```python
from build123d import *

# Parameters (mm, degrees)
SKETCH1_W           = 42.3
SKETCH1_H           = 42.3
BOSS_EXTRUDE1_DEPTH = 3
SKETCH2_R           = 1.5
CUT_EXTRUDE1_DEPTH  = 4
SKETCH5_W           = 3
SKETCH5_H           = 42.3
BOSS_EXTRUDE2_DEPTH = 40
CUT_EXTRUDE2_DEPTH  = 40
SKETCH7_R           = 1.5
CUT_EXTRUDE3_DEPTH  = 4


with BuildPart() as part:
    # Sketch1 → Boss-Extrude1 (new body)
    with BuildSketch(Plane(origin=(0, 0, 0), x_dir=(1, 0, 0), z_dir=(0, 1, 0))):
        with Locations((21.15, 21.15)):
            Rectangle(SKETCH1_W, SKETCH1_H)
    extrude(amount=BOSS_EXTRUDE1_DEPTH)

    # Sketch2 → Cut-Extrude1 (cut, through all)
    with BuildSketch(Plane(origin=(0, 3, 0), x_dir=(1, 0, 0), z_dir=(0, 1, 0))):
        with Locations((5.65, 5.65)):
            Circle(SKETCH2_R)
        with Locations((36.65, 5.65)):
            Circle(SKETCH2_R)
        with Locations((36.65, 36.65)):
            Circle(SKETCH2_R)
        with Locations((5.65, 36.65)):
            Circle(SKETCH2_R)
    extrude(amount=-CUT_EXTRUDE1_DEPTH, mode=Mode.SUBTRACT)

    # Sketch5 → Boss-Extrude2 (add)
    with BuildSketch(Plane(origin=(0, 3, 0), x_dir=(1, 0, 0), z_dir=(0, 1, 0))):
        with Locations((40.8, 21.15)):
            Rectangle(SKETCH5_W, SKETCH5_H)
    extrude(amount=BOSS_EXTRUDE2_DEPTH)

    # Sketch6 → Cut-Extrude2 (cut)
    with BuildSketch(Plane.ZY.offset(-39.3)):
        Polygon((-42.3, 43), (-22.3, 43), (-42.3, 23), align=None)
    extrude(amount=-CUT_EXTRUDE2_DEPTH, mode=Mode.SUBTRACT)

    # Sketch7 → Cut-Extrude3 (cut, through all)
    with BuildSketch(Plane.ZY.offset(-39.3)):
        with Locations((-10, 33)):
            Circle(SKETCH7_R)
        with Locations((-10, 13)):
            Circle(SKETCH7_R)
    extrude(amount=-CUT_EXTRUDE3_DEPTH, mode=Mode.SUBTRACT)


solid = part.part
```
Can you work these out from the model? Positions are in its coordinate system, mm. A direction names the side the tool comes from. Coordinates: 2 decimals unless noted, no trailing zeros. Order: outer loops, then holes, each group sorted by start corner. A loop starts at its lowest first (then second) coordinate and runs counter-clockwise, first axis right, second up. Notation, with made-up numbers: (13.5, -10.5) - (49.5, -10.5) arc R17 cw to (49.5, 16.5) - close; hole circle Ø8 at (84, 7). An arc over 180 degrees is marked (long way). Answer in a Markdown table with one row per item.
1. Suppose I cut it at C-C (y = 13). Please give me the cut outline in (x, z).
Reply:
| item | result |
|---|---|
| outline | (39.3, -42.3) - (42.3, -42.3) - (42.3, -11.5) - (39.3, -11.5) - close; (39.3, -8.5) - (42.3, -8.5) - (42.3, 0) - (39.3, 0) - close |
2. If we mould it in two halves opening along X, with no side actions, what happens to faces 3 (the flat face through (30, 2, 0)), 4 (the cylindrical face through (38.08, 1.52, -6.1)), 5 (the flat face through (0, 1, -21))? For each: pulls with the +X half, pulls with the -X half, needs draft (parallel to the pull), parting line crosses it, or undercut.
Reply:
| item | result |
|---|---|
| face 3 | needs draft |
| face 4 | undercut |
| face 5 | pulls with the -X half |
3. If I drill on line 1 along Y through (x, z) = (40.4, -10); line 2 along Z through (x, y) = (36.65, 2.25); line 3 along X through (y, z) = (2.3, -5.65), over which ranges is the centre line in solid material (lowest first)?
Reply:
| item | result |
|---|---|
| line 1 | y = 0 to 11.5, 14.5 to 31.5, 34.5 to 43 |
| line 2 | z = -42.3 to -38.15, -35.15 to -7.15, -4.15 to 0 |
| line 3 | x = 0 to 4.15, 7.15 to 35.15, 38.15 to 42.3 |
4. For pin 1 (5 mm diameter, centred on y = 33, z = -10, fed in from +X); pin 2 (4 mm diameter, centred on x = 36.65, z = -36.65, fed in from +Y); pin 3 (10 mm diameter, centred on y = 29.5, z = -15.5, fed in from -X), each with a flat end and sliding along its axis, tell me the tip position at first contact or that it passes through.
Reply:
| item | result |
|---|---|
| pin 1 | stops at x = 42.3 |
| pin 2 | stops at y = 3 |
| pin 3 | stops at x = 39.3 |
5. Suppose I cut it at B-B (x = 36.65). Please give me the cut outline in (y, z).
Reply:
| item | result |
|---|---|
| outline | (0, -42.3) - (3, -42.3) - (3, -38.15) - (0, -38.15) - close; (0, -35.15) - (3, -35.15) - (3, -7.15) - (0, -7.15) - close; (0, -4.15) - (3, -4.15) - (3, 0) - (0, 0) - close |
6. Suppose I cut it at D-D (z = -34). Please give me the cut outline in (x, y).
Reply:
| item | result |
|---|---|
| outline | (0, 0) - (42.3, 0) - (42.3, 31.3) - (39.3, 31.3) - (39.3, 3) - (0, 3) - close |
7. For faces 1 (the flat face through (39.3, 23, -21)), 2 (the flat face through (26, 2, -42.3)), which set-ups out of +Z, -Z, +X, -X, +Y, -Y let a thin tool reach every point of the face, with its end or its side?
Reply:
| item | result |
|---|---|
| face 1 | +Z, -Z, -X, +Y |
| face 2 | -Z, +X, -X, +Y, -Y |
8. Suppose I cut it at A-A (z = -5.65). Please give me the cut outline in (x, y), and give its area (3 significant figures).
Reply:
| item | result |
|---|---|
| outline | (0, 0) - (4.15, 0) - (4.15, 3) - (0, 3) - close; (7.15, 0) - (35.15, 0) - (35.15, 3) - (7.15, 3) - close; (38.15, 0) - (42.3, 0) - (42.3, 43) - (39.3, 43) - (39.3, 3) - (38.15, 3) - close |
| area | 229 mm^2 |
